```python
from build123d import *

# Parameters (mm, degrees)
SKETCH1_W           = 116.84
SKETCH1_H           = 88.9
BOSS_EXTRUDE1_DEPTH = 30.48
SKETCH2_W           = 121.92
SKETCH2_H           = 60.96
CUT_EXTRUDE1_DEPTH  = 15.24
SKETCH4_W           = 38.1
SKETCH4_H           = 30.48
CUT_EXTRUDE2_DEPTH  = 25.4
SKETCH9_W           = 2.54
SKETCH9_H           = 60.96
BOSS_EXTRUDE2_DEPTH = 15.24
SKETCH11_W          = 2.54
SKETCH11_H          = 60.96
BOSS_EXTRUDE3_DEPTH = 15.24
SKETCH13_W          = 6.933470389
SKETCH13_H          = 38.1
CUT_EXTRUDE6_DEPTH  = 15.24
SKETCH14_W          = 5.795170267
SKETCH14_H          = 19.05
CUT_EXTRUDE7_DEPTH  = 15.24
SKETCH15_R          = 1.905
CUT_EXTRUDE8_DEPTH  = 48.26
SKETCH16_R          = 1.905
CUT_EXTRUDE9_DEPTH  = 6.858
SKETCH19_W          = 52.412757742
SKETCH19_H          = 17.024597759
CUT_EXTRUDE10_DEPTH = 4.233333333
SKETCH5_W           = 10.150117587
SKETCH5_H           = 22.048837971
CUT_EXTRUDE3_DEPTH  = 15.24
SKETCH6_W           = 9.22767553
SKETCH6_H           = 28.682463558
CUT_EXTRUDE4_DEPTH  = 15.24
SKETCH7_W           = 7.203031043
SKETCH7_H           = 12.7
CUT_EXTRUDE5_DEPTH  = 15.24


with BuildPart() as part:
    # Sketch1 → Boss-Extrude1 (new body)
    with BuildSketch(Plane.XY):
        Rectangle(SKETCH1_W, SKETCH1_H)
    extrude(amount=BOSS_EXTRUDE1_DEPTH)

    # Sketch2 → Cut-Extrude1 (cut)
    with BuildSketch(Plane.XY):
        with Locations((0, 11.43)):
            Rectangle(SKETCH2_W, SKETCH2_H)
    extrude(amount=CUT_EXTRUDE1_DEPTH, mode=Mode.SUBTRACT)

    # Sketch4 → Cut-Extrude2 (cut)
    with BuildSketch(Plane(origin=(0, 0, 0), x_dir=(-1, 0, 0), z_dir=(0, 0, -1))):
        with Locations((-27.432, -24.13)):
            Rectangle(SKETCH4_W, SKETCH4_H)
    extrude(amount=-CUT_EXTRUDE2_DEPTH, mode=Mode.SUBTRACT)

    # Sketch9 → Boss-Extrude2 (add)
    with BuildSketch(Plane(origin=(0, 0, 15.24), x_dir=(-1, 0, 0), z_dir=(0, 0, -1))):
        with Locations((-57.15, 11.43)):
            Rectangle(SKETCH9_W, SKETCH9_H)
    extrude(amount=BOSS_EXTRUDE2_DEPTH)

    # Sketch11 → Boss-Extrude3 (add)
    with BuildSketch(Plane(origin=(0, 0, 15.24), x_dir=(-1, 0, 0), z_dir=(0, 0, -1))):
        with Locations((57.15, 11.43)):
            Rectangle(SKETCH11_W, SKETCH11_H)
    extrude(amount=BOSS_EXTRUDE3_DEPTH)

    # Sketch13 → Cut-Extrude6 (cut)
    with BuildSketch(Plane(origin=(0, 0, 0), x_dir=(-1, 0, 0), z_dir=(0, 0, -1))):
        with Locations((59.346735194, 12.7)):
            Rectangle(SKETCH13_W, SKETCH13_H)
    extrude(amount=-CUT_EXTRUDE6_DEPTH, mode=Mode.SUBTRACT)

    # Sketch14 → Cut-Extrude7 (cut)
    with BuildSketch(Plane(origin=(0, 0, 0), x_dir=(-1, 0, 0), z_dir=(0, 0, -1))):
        with Locations((-58.777585134, 32.385)):
            Rectangle(SKETCH14_W, SKETCH14_H)
    extrude(amount=-CUT_EXTRUDE7_DEPTH, mode=Mode.SUBTRACT)

    # Sketch15 → Cut-Extrude8 (cut)
    with BuildSketch(Plane(origin=(0, 0, 15.24), x_dir=(-1, 0, 0), z_dir=(0, 0, -1))):
        with Locations((52.07, 36.068)):
            Circle(SKETCH15_R)
        with Locations((52.07, -12.7)):
            Circle(SKETCH15_R)
        with Locations((-52.07, 15.748)):
            Circle(SKETCH15_R)
    extrude(amount=-CUT_EXTRUDE8_DEPTH, mode=Mode.SUBTRACT)

    # Sketch16 → Cut-Extrude9 (cut)
    with BuildSketch(Plane(origin=(0, 0, 0), x_dir=(-1, 0, 0), z_dir=(0, 0, -1))):
        with Locations((-52.451, -23.8506)):
            Circle(SKETCH16_R)
        with Locations((-2.413, -23.8506)):
            Circle(SKETCH16_R)
    extrude(amount=-CUT_EXTRUDE9_DEPTH, mode=Mode.SUBTRACT)

    # Sketch19 → Cut-Extrude10 (cut)
    with BuildSketch(Plane(origin=(0, 0, 0), x_dir=(-1, 0, 0), z_dir=(0, 0, -1))):
        with Locations((29.681257837, -30.857701121)):
            Rectangle(SKETCH19_W, SKETCH19_H)
    extrude(amount=-CUT_EXTRUDE10_DEPTH, mode=Mode.SUBTRACT)

    # Sketch5 → Cut-Extrude3 (cut)
    with BuildSketch(Plane(origin=(0, 0, 0), x_dir=(-1, 0, 0), z_dir=(0, 0, -1))):
        with Locations((66.035058793, 15.645581015)):
            Rectangle(SKETCH5_W, SKETCH5_H)
    extrude(amount=-CUT_EXTRUDE3_DEPTH, mode=Mode.SUBTRACT)

    # Sketch6 → Cut-Extrude4 (cut)
    with BuildSketch(Plane(origin=(0, 0, 0), x_dir=(-1, 0, 0), z_dir=(0, 0, -1))):
        with Locations((65.573837765, 15.522274396)):
            Rectangle(SKETCH6_W, SKETCH6_H)
    extrude(amount=-CUT_EXTRUDE4_DEPTH, mode=Mode.SUBTRACT)

    # Sketch7 → Cut-Extrude5 (cut)
    with BuildSketch(Plane(origin=(0, 0, 0), x_dir=(-1, 0, 0), z_dir=(0, 0, -1))):
        with Locations((-64.561515521, 35.56)):
            Rectangle(SKETCH7_W, SKETCH7_H)
    extrude(amount=-CUT_EXTRUDE5_DEPTH, mode=Mode.SUBTRACT)


solid = part.part
```
Model file for the job. Use its own axes, mm. A direction names the side the tool comes from. Coordinates: 2 decimals unless noted, no trailing zeros. Order: outer loops, then holes, each group sorted by start corner. A loop starts at its lowest first (then second) coordinate and runs counter-clockwise, first axis right, second up. Notation, with made-up numbers: (21.25, -0.5) - (61.25, -0.5) arc R20 ccw to (61.25, 26.5) - close; hole circle Ø10 at (55, 53). An arc over 180 degrees is marked (long way). Return JSON: item names as keys, results as strings. Group by question number.
1) Saw through at B-B, the plane y = -12.7. Write the cut outline in (x, z) (3 decimals), plus the area to 3 significant figures.
2) Flat gauge pins, fed straight in: P1, Ø8, axis at y = 37.5, z = 10.5, coming from the +X side; P2, Ø15, axis at x = 31, y = -28.5, coming from the -Z side. Where does each tip first touch, or does it go through?
3) Tool access for faces 5 (the flat face through (52, -24, 6.858)), 6 (the cylindrical face through (51.046, 17.354, 22.753)): list every direction of +Z, -Z, +X, -X, +Y, -Y with a clear straight run to the whole face (end or side of a thin tool).
4) Mould opens along X. For faces 1 (the flat face through (-58.42, -1, 19)), 2 (the flat face through (-24, -19.05, 8)), 3 (the flat face through (-55.88, 37, 8)), 4 (the flat face through (-57, -6.35, 8)) say: released by +X, released by -X, zero draft, split by the parting line, or undercut.
5) Saw through at D-D, the plane y = -30. Write the cut outline in (x, z), plus the area to 3 significant figures.
6) Saw through at A-A, the plane x = -52.07. Write the cut outline in (y, z) (3 decimals), plus the area to 3 significant figures.
7) Probe line 1 (X direction, y = -36, z = 2.5); line 2 (Y direction, x = -52.07, z = 27) (3 decimals); line 3 (X direction, y = -34.5, z = 13.5). List the from-to ranges inside material, lowest first. Write a range as from..to.
8) Saw through at C-C, the plane x = 34. Write the cut outline in (y, z), plus the area to 3 significant figures.
Values found:
{
 "1": {"outline": "(-58.42, 0) - (-55.88, 0) - (-55.88, 15.24) - (-53.975, 15.24) - (-53.975, 30.48) - (-58.42, 30.48) - close; (-50.165, 15.24) - (8.382, 15.24) - (8.382, 25.4) - (46.482, 25.4) - (46.482, 15.24) - (55.88, 15.24) - (55.88, 0) - (58.42, 0) - (58.42, 30.48) - (-50.165, 30.48) - close", "area": "1,410 mm²"},
 "2": {"P1": "stops at x = -55.88", "P2": "stops at z = 25.4"},
 "3": {"face 5": "-Z", "face 6": "+Z, -Z"},
 "4": {"face 1": "released by -X", "face 2": "undercut", "face 3": "released by +X", "face 4": "zero draft"},
 "5": {"outline": "(-58.42, 0) - (-55.89, 0) - (-55.89, 4.23) - (-3.47, 4.23) - (-3.47, 0) - (8.38, 0) - (8.38, 25.4) - (46.48, 25.4) - (46.48, 0) - (58.42, 0) - (58.42, 30.48) - (-58.42, 30.48) - close", "area": "2,370 mm²"},
 "6": {"outline": "(-44.45, 0) - (-39.37, 0) - (-39.37, 4.233) - (-22.345, 4.233) - (-22.345, 0) - (-19.05, 0) - (-19.05, 15.24) - (-14.605, 15.24) - (-14.605, 30.48) - (-44.45, 30.48) - close; (-10.795, 15.24) - (34.163, 15.24) - (34.163, 30.48) - (-10.795, 30.48) - close; (37.973, 15.24) - (41.91, 15.24) - (41.91, 0) - (44.45, 0) - (44.45, 30.48) - (37.973, 30.48) - close", "area": "1,590 mm²"},
 "7": {"line 1": "x = -58.42..-55.89, -3.47..8.38, 46.48..58.42", "line 2": "y = -44.45..-14.605, -10.795..34.163, 37.973..44.45", "line 3": "x = -58.42..8.38, 46.48..58.42"},
 "8": {"outline": "(-44.45, 0) - (-39.37, 0) - (-39.37, 25.4) - (-8.89, 25.4) - (-8.89, 15.24) - (41.91, 15.24) - (41.91, 0) - (44.45, 0) - (44.45, 30.48) - (-44.45, 30.48) - close", "area": "1,160 mm²"}
}
